Verification items for the finished model (mm, model axes). A direction names the side the tool comes from. Give positions to 0.01 mm unless a question says otherwise; leave off trailing zeros. Loops run counter-clockwise (first coordinate to the right, second up) from the corner with the lowest first, then second, coordinate; pieces in that order, holes last. Notation, with made-up numbers: (7.5, 33) - (28.5, 33) arc R7 ccw to (28.5, 41) - close; hole circle Ø2 at (36.25, -4.5). An arc over 180 degrees is marked (long way). Put each result on its own line as item: value. Start each with the question number.
```python
from build123d import *

# Parameters (mm, degrees)
SKETCH1_R           = 6.15
SKETCH1_R_2         = 5.35
SKETCH1_R_3         = 2.75
BOSS_EXTRUDE1_DEPTH = 1.9
SKETCH1_3_R         = 5.35
SKETCH1_3_R_2       = 2.75
BOSS_EXTRUDE2_DEPTH = 14.4
SKETCH2_R           = 2.75
SKETCH2_R_2         = 1.9
SKETCH2_R_3         = 1.15
SKETCH2_R_4         = 0.85
BOSS_EXTRUDE3_DEPTH = 3
SKETCH2_3_R         = 1.15
SKETCH2_3_R_2       = 0.85
SKETCH2_3_R_3       = 1.9
BOSS_EXTRUDE4_DEPTH = 0.8
SKETCH2_5_R         = 0.85
BOSS_EXTRUDE5_DEPTH = 14
SKETCH2_6_R         = 1.15
SKETCH2_6_R_2       = 0.85
BOSS_EXTRUDE6_DEPTH = 5.2
SKETCH2_7_W         = 3
SKETCH2_7_H         = 0.2
BOSS_EXTRUDE7_DEPTH = 9.6


with BuildPart() as part:
    # Sketch1 → Boss-Extrude1 (new body)
    with BuildSketch(Plane.XY):
        Circle(SKETCH1_R)
        Circle(SKETCH1_R_2, mode=Mode.SUBTRACT)
        Circle(SKETCH1_R_2)
        Circle(SKETCH1_R_3, mode=Mode.SUBTRACT)
    extrude(amount=BOSS_EXTRUDE1_DEPTH)

    # Sketch1_3 → Boss-Extrude2 (add)
    with BuildSketch(Plane.XY):
        Circle(SKETCH1_3_R)
        Circle(SKETCH1_3_R_2, mode=Mode.SUBTRACT)
    extrude(amount=-BOSS_EXTRUDE2_DEPTH)

    # Sketch2 → Boss-Extrude3 (add)
    with BuildSketch(Plane(origin=(0, 0, -14.4), x_dir=(-1, 0, 0), z_dir=(0, 0, -1))):
        Circle(SKETCH2_R)
        Circle(SKETCH2_R_2, mode=Mode.SUBTRACT)
        Circle(SKETCH2_R_2)
        Circle(SKETCH2_R_3, mode=Mode.SUBTRACT)
        Circle(SKETCH2_R_3)
        Circle(SKETCH2_R_4, mode=Mode.SUBTRACT)
        Circle(SKETCH2_R_4)
    extrude(amount=-BOSS_EXTRUDE3_DEPTH)

    # Sketch2_3 → Boss-Extrude4 (add)
    with BuildSketch(Plane(origin=(0, 0, -14.4), x_dir=(-1, 0, 0), z_dir=(0, 0, -1))):
        Circle(SKETCH2_3_R)
        Circle(SKETCH2_3_R_2, mode=Mode.SUBTRACT)
        Circle(SKETCH2_3_R_2)
        Circle(SKETCH2_3_R_3)
        Circle(SKETCH2_3_R, mode=Mode.SUBTRACT)
    extrude(amount=BOSS_EXTRUDE4_DEPTH)

    # Sketch2_5 → Boss-Extrude5 (add)
    with BuildSketch(Plane(origin=(0, 0, -14.4), x_dir=(-1, 0, 0), z_dir=(0, 0, -1))):
        Circle(SKETCH2_5_R)
    extrude(amount=-BOSS_EXTRUDE5_DEPTH)

    # Sketch2_6 → Boss-Extrude6 (add)
    with BuildSketch(Plane(origin=(0, 0, -14.4), x_dir=(-1, 0, 0), z_dir=(0, 0, -1))):
        Circle(SKETCH2_6_R)
        Circle(SKETCH2_6_R_2, mode=Mode.SUBTRACT)
        Circle(SKETCH2_6_R_2)
    extrude(amount=BOSS_EXTRUDE6_DEPTH)

    # Sketch2_7 → Boss-Extrude7 (add)
    with BuildSketch(Plane(origin=(0, 0, -14.4), x_dir=(-1, 0, 0), z_dir=(0, 0, -1))):
        with Locations((0, 5.035416244)):
            Rectangle(SKETCH2_7_W, SKETCH2_7_H)
    extrude(amount=BOSS_EXTRUDE7_DEPTH)


solid = part.part
```
1) Depth check by flat-ended pin: P1, Ø1, axis at y = 4, z = -9, coming from the -X side; P2, Ø5, axis at x = -3.5, z = -13.5, coming from the -Y side; P3, Ø1.4, axis at x = -0.5, y = 0.5, coming from the +Z side. Enter the tip coordinate at first touch or a pass-through.
2) Scan lines: line 1 along Y through (x, z) = (0, -4.5); line 2 along Y through (x, z) = (0.5, -8.25); line 3 along Z through (x, y) = (4.75, -1.75). Record each from-to range of solid material in increasing order. Write a range as from..to.
3) Section check A-A, the plane z = -9.5. Enter the section's corners in (x, y), plus the area to 3 significant figures.
4) Section check D-D, the plane y = 0. Enter the section's corners in (x, z), plus the area to 3 significant figures.
5) Draft check along X on faces 5 (the face through (0, 0, -19.6)), 6 (the face through (-0.596, -2.685, -4.843)), 7 (the face through (1, -1, -11.4)), 8 (the face through (1.9, 0.08, -14.79)). Enter one of: pulls with the +X half, pulls with the -X half, needs draft (parallel to the pull), parting line crosses it, or undercut.
6) Set-up check for faces 1 (the face through (0.18, -0.83, -5.98)), 2 (the face through (0.91, -0.7, -17.37)), 3 (the face through (0, 5.135, -19)), 4 (the face through (0, 4.935, -19)): record each of +Z, -Z, +X, -X, +Y, -Y from which the full face is reachable in a straight line by a thin tool's end or side.
7) Section check C-C, the plane z = -18. Enter the section's corners in (x, y).
8) Section check B-B, the plane x = 0. Enter the section's corners in (y, z), plus the area to 3 significant figures.
Results are:
1. P1: stops at x = -4.05
1. P2: stops at y = -5.26
1. P3: stops at z = -0.4
2. line 1: y = -5.35..-2.75, -0.85..0.85, 2.75..5.35
2. line 2: y = -5.33..-2.7, -0.69..0.69, 2.7..5.33
2. line 3: z = -14.4..1.9
3. outline: circle Ø10.7 at (0, 0); circle Ø1.7 at (0, 0); hole circle Ø5.5 at (0, 0)
3. area: 68.4 mm2
4. outline: (-6.15, 0) - (-5.35, 0) - (-5.35, -14.4) - (-1.9, -14.4) - (-1.9, -15.2) - (-1.15, -15.2) - (-1.15, -19.6) - (1.15, -19.6) - (1.15, -15.2) - (1.9, -15.2) - (1.9, -14.4) - (5.35, -14.4) - (5.35, 0) - (6.15, 0) - (6.15, 1.9) - (2.75, 1.9) - (2.75, -11.4) - (0.85, -11.4) - (0.85, -0.4) - (-0.85, -0.4) - (-0.85, -11.4) - (-2.75, -11.4) - (-2.75, 1.9) - (-6.15, 1.9) - close
4. area: 136 mm2
5. face 5: needs draft
5. face 6: undercut
5. face 7: undercut
5. face 8: parting line crosses it
6. face 1: +Z
6. face 2: -Z
6. face 3: -Z, +X, -X, +Y
6. face 4: -Z, +X, -X
7. outline: (-1.5, 4.94) - (1.5, 4.94) - (1.5, 5.14) - (-1.5, 5.14) - close; circle Ø2.3 at (0, 0)
8. outline: (-6.15, 0) - (-5.35, 0) - (-5.35, -14.4) - (-1.9, -14.4) - (-1.9, -15.2) - (-1.15, -15.2) - (-1.15, -19.6) - (1.15, -19.6) - (1.15, -15.2) - (1.9, -15.2) - (1.9, -14.4) - (4.94, -14.4) - (4.94, -24) - (5.14, -24) - (5.14, -14.4) - (5.35, -14.4) - (5.35, 0) - (6.15, 0) - (6.15, 1.9) - (2.75, 1.9) - (2.75, -11.4) - (0.85, -11.4) - (0.85, -0.4) - (-0.85, -0.4) - (-0.85, -11.4) - (-2.75, -11.4) - (-2.75, 1.9) - (-6.15, 1.9) - close
8. area: 138 mm2
